Study the drawing (mm; zero at the part's minimum x, y, z) and answer. A direction names the side the tool comes from. Give positions to 0.01 mm unless a question says otherwise; leave off trailing zeros. Order: outer loops, then holes, each group sorted by start corner. A loop starts at its lowest first (then second) coordinate and runs counter-clockwise, first axis right, second up. Notation, with made-up numbers: (22.5, 46.25) - (42.5, 46.25) arc R30 ccw to (42.5, 68.25) - close; hole circle Ø9 at (-2, 81.5). An arc over 180 degrees is marked (long way). Return JSON: item names as keys, results as strings.
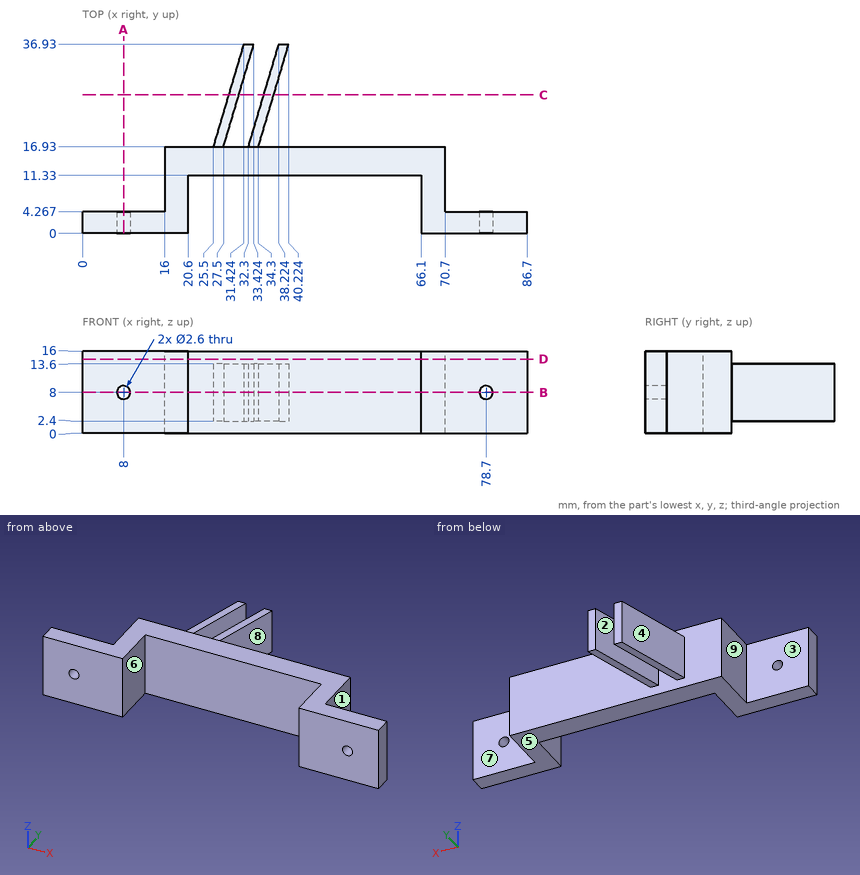
Q1. For the marked faces 5, 6, 7, 8 and 9, determine the directions among +Z, -Z, +X, -X, +Y, -Y from which every point of the face is accessible in a straight line to the end or side of a thin tool.
Values:
{"face 5": "-Z, +X, -X, +Y, -Y", "face 6": "+Z, -Z, -Y", "face 7": "+Z, -Z, +X, +Y", "face 8": "+Z, -Z, +X", "face 9": "+Z, -Z, -X, +Y"}
Q2. Determine the mould class of the marked faces 1, 2, 3 and 4 for opening direction X: released by +X, released by -X, zero draft, split by the parting line, or undercut.
Values:
{"face 1": "released by +X", "face 2": "undercut", "face 3": "zero draft", "face 4": "released by -X"}
Q3. A cutting plane is placed at C-C (y = 27). Write down the section's boundary in (x, z).
Values:
{"outline": "(28.48, 2.4) - (30.48, 2.4) - (30.48, 13.6) - (28.48, 13.6) - close; (35.28, 2.4) - (37.28, 2.4) - (37.28, 13.6) - (35.28, 13.6) - close"}
Q4. Given pin 1 (4 mm diameter, centred on x = 29.5, y = 28.5, fed in from +Z); pin 2 (4 mm diameter, centred on x = 28.5, z = 13.5, fed in from -Y); pin 3 (8 mm diameter, centred on x = 47, z = 4.5, fed in from +Y), each flat-ended and moving along its own axis, determine where each tip first touches the part or whether it passes through.
Values:
{"pin 1": "stops at z = 13.6", "pin 2": "stops at y = 11.33", "pin 3": "stops at y = 16.93"}
Q5. A cutting plane is placed at A-A (x = 8). Write down the section's boundary in (y, z).
Values:
{"outline": "(0, 0) - (4.27, 0) - (4.27, 6.7) - (0, 6.7) - close; (0, 9.3) - (4.27, 9.3) - (4.27, 16) - (0, 16) - close"}
Q6. A cutting plane is placed at D-D (z = 14.5). Write down the section's boundary in (x, y), and give its area (3 significant figures).
Values:
{"outline": "(0, 0) - (20.6, 0) - (20.6, 11.33) - (66.1, 11.33) - (66.1, 0) - (86.7, 0) - (86.7, 4.27) - (70.7, 4.27) - (70.7, 16.93) - (16, 16.93) - (16, 4.27) - (0, 4.27) - close", "area": "547 mm²"}
Q7. A cutting plane is placed at B-B (z = 8). Write down the section's boundary in (x, y), and give its area (3 significant figures).
Values:
{"outline": "(0, 0) - (6.7, 0) - (6.7, 4.27) - (0, 4.27) - close; (9.3, 0) - (20.6, 0) - (20.6, 11.33) - (66.1, 11.33) - (66.1, 0) - (77.4, 0) - (77.4, 4.27) - (70.7, 4.27) - (70.7, 16.93) - (34.3, 16.93) - (40.22, 36.93) - (38.22, 36.93) - (32.3, 16.93) - (27.5, 16.93) - (33.42, 36.93) - (31.42, 36.93) - (25.5, 16.93) - (16, 16.93) - (16, 4.27) - (9.3, 4.27) - close; (80, 0) - (86.7, 0) - (86.7, 4.27) - (80, 4.27) - close", "area": "605 mm²"}
Q8. Consider L1, parallel to X at y = 1, z = 8; L2, parallel to Z at x = 8, y = 2.15; L3, parallel to X at y = 16, z = 13.25. Determine where each line is inside the solid, lowest interval first.
Values:
{"L1": "x = 0 to 6.7, 9.3 to 20.6, 66.1 to 77.4, 80 to 86.7", "L2": "z = 0 to 6.7, 9.3 to 16", "L3": "x = 16 to 70.7"}
